from build123d import *
from build123d.topology import SkipClean

# Parameters (mm, degrees)
SKETCH_1_W          = 50
SKETCH_1_H          = 15
SKETCH_1_R          = 1.1
SKETCH_1_R_2        = 1.5
SKETCH_1_R_3        = 2.6
EXTRUDE_1_DEPTH     = 2
SKETCH_3_R          = 3
CUT_EXTRUDE_1_DEPTH = 1.5
SKETCH_1_7_W        = 17
SKETCH_1_7_H        = 15
SKETCH_1_7_R        = 1.5
SKETCH_1_7_R_2      = 1.1
EXTRUDE_4_DEPTH     = 4
SKETCH_1_8_R        = 6
SKETCH_1_8_R_2      = 1.5
SKETCH_1_8_R_3      = 1.1
CUT_EXTRUDE_4_DEPTH = 2
CUT_EXTRUDE_5_DEPTH = 15
EXTRUDE_START       = 2
SKETCH_8_R          = 5.5
SKETCH_8_R_2        = 2.6
EXTRUDE_11_DEPTH    = 2
CUT_EXTRUDE_6_DEPTH = 3.5
CUT_EXTRUDE_7_DEPTH = 2
FILLET_1_R          = 2
EXTRUDE_15_DEPTH    = 1
EXTRUDE_16_DEPTH    = 2
SKETCH_16_R         = 4.1
SKETCH_16_R_2       = 2.6
EXTRUDE_18_DEPTH    = 5
FILLET_3_R          = 0.5


with BuildPart() as part:
    # 草图1 → 凸台-拉伸1 (new body)
    with BuildSketch(Plane(origin=(0, 0, 0), x_dir=(1, 0, 0), z_dir=(0, 1, 0))):
        Rectangle(SKETCH_1_W, SKETCH_1_H)
        with BuildLine():
            ThreePointArc((8, 2.598076211), (8.5, 0), (8, -2.598076211))
            Line((8, -2.598076211), (8, 2.598076211))
        make_face(mode=Mode.SUBTRACT)
        with Locations(Location((-19.330127019, -2.5, 0), (0, 0, 270))):
            Circle(SKETCH_1_R, mode=Mode.SUBTRACT)
        with Locations(Location((-15, 0, 0), (0, 0, 270))):
            Circle(SKETCH_1_R_2, mode=Mode.SUBTRACT)
        with Locations(Location((-10.669872981, 2.5, 0), (0, 0, 270))):
            Circle(SKETCH_1_R, mode=Mode.SUBTRACT)
        with Locations(Location((1.5, 0, 0), (0, 0, 270))):
            Circle(SKETCH_1_R_3, mode=Mode.SUBTRACT)
        with Locations(Location((17.5, 3.5, 0), (0, 0, 270))):
            Circle(SKETCH_1_R, mode=Mode.SUBTRACT)
        with Locations(Location((17.5, -3.5, 0), (0, 0, 270))):
            Circle(SKETCH_1_R, mode=Mode.SUBTRACT)
        with Locations(Location((14, 0, 0), (0, 0, 270))):
            Circle(SKETCH_1_R, mode=Mode.SUBTRACT)
        with Locations(Location((17.5, 0, 0), (0, 0, 270))):
            Circle(SKETCH_1_R_2, mode=Mode.SUBTRACT)
        with Locations(Location((21, 0, 0), (0, 0, 270))):
            Circle(SKETCH_1_R, mode=Mode.SUBTRACT)
    extrude(amount=EXTRUDE_1_DEPTH)

    # 草图3 → 切除-拉伸1 (cut)
    with BuildSketch(Plane.XZ):
        with Locations(Location((-15, 0, 0), (0, 0, 270))):
            Circle(SKETCH_3_R)
    extrude(amount=-CUT_EXTRUDE_1_DEPTH, mode=Mode.SUBTRACT)

    # 草图1<7> → 凸台-拉伸4 (add)
    with BuildSketch(Plane(origin=(0, 0, 0), x_dir=(1, 0, 0), z_dir=(0, 1, 0))):
        with Locations((16.5, 0)):
            Rectangle(SKETCH_1_7_W, SKETCH_1_7_H)
        with Locations(Location((17.5, 0, 0), (0, 0, 270))):
            Circle(SKETCH_1_7_R, mode=Mode.SUBTRACT)
        with Locations(Location((21, 0, 0), (0, 0, 270))):
            Circle(SKETCH_1_7_R_2, mode=Mode.SUBTRACT)
        with Locations(Location((17.5, -3.5, 0), (0, 0, 270))):
            Circle(SKETCH_1_7_R_2, mode=Mode.SUBTRACT)
        with Locations(Location((14, 0, 0), (0, 0, 270))):
            Circle(SKETCH_1_7_R_2, mode=Mode.SUBTRACT)
        with Locations(Location((17.5, 3.5, 0), (0, 0, 270))):
            Circle(SKETCH_1_7_R_2, mode=Mode.SUBTRACT)
    extrude(amount=EXTRUDE_4_DEPTH)

    # 草图1<8> → 切除-拉伸4 (cut)
    with BuildSketch(Plane(origin=(0, 0, 0), x_dir=(1, 0, 0), z_dir=(0, 1, 0))):
        with Locations(Location((17.5, 0, 0), (0, 0, 270))):
            Circle(SKETCH_1_8_R)
        with Locations(Location((17.5, 0, 0), (0, 0, 270))):
            Circle(SKETCH_1_8_R_2, mode=Mode.SUBTRACT)
        with Locations(Location((21, 0, 0), (0, 0, 270))):
            Circle(SKETCH_1_8_R_3, mode=Mode.SUBTRACT)
        with Locations(Location((17.5, -3.5, 0), (0, 0, 270))):
            Circle(SKETCH_1_8_R_3, mode=Mode.SUBTRACT)
        with Locations(Location((14, 0, 0), (0, 0, 270))):
            Circle(SKETCH_1_8_R_3, mode=Mode.SUBTRACT)
        with Locations(Location((17.5, 3.5, 0), (0, 0, 270))):
            Circle(SKETCH_1_8_R_3, mode=Mode.SUBTRACT)
    extrude(amount=CUT_EXTRUDE_4_DEPTH, mode=Mode.SUBTRACT)

    # 草图6 → 切除-拉伸5 (cut)
    with BuildSketch(Plane(origin=(0, 0, -7.5), x_dir=(-1, 0, 0), z_dir=(0, 0, -1))):
        Polygon((-8, 2), (-11.464101615, 4), (-8, 4), align=None)
    extrude(amount=-CUT_EXTRUDE_5_DEPTH, mode=Mode.SUBTRACT)

    # 草图8 → 凸台-拉伸11 (add)
    with SkipClean():  # the faces are left unmerged after this step: merging them gives an invalid solid
        with BuildSketch(Plane.XZ.offset(EXTRUDE_START)):
            with Locations(Location((1.5, 0, 0), (0, 0, 90))):
                Circle(SKETCH_8_R)
            with Locations(Location((1.5, 0, 0), (0, 0, 270))):
                Circle(SKETCH_8_R_2, mode=Mode.SUBTRACT)
        extrude(amount=-EXTRUDE_11_DEPTH)

    # 草图10 → 切除-拉伸6 (cut)
    with BuildSketch(Plane.XZ.offset(2)):
        Polygon((1.5, 3.175426481), (-1.25, 1.58771324), (-1.25, -1.58771324), (1.5, -3.175426481), (4.25, -1.58771324), (4.25, 1.58771324), align=None)
    extrude(amount=-CUT_EXTRUDE_6_DEPTH, mode=Mode.SUBTRACT)

    # 草图11 → 切除-拉伸7 (cut)
    with BuildSketch(Plane.XZ.offset(2)):
        with BuildLine():
            Line((-3.398979486, 2.5), (6.398979486, 2.5))
            ThreePointArc((6.398979486, 2.5), (1.5, 5.5), (-3.398979486, 2.5))
        make_face()
    extrude(amount=-CUT_EXTRUDE_7_DEPTH, mode=Mode.SUBTRACT)

    # 圆角1
    fillet_1_edges = [part.edges().sort_by_distance(p)[0] for p in [
        (-25, 1, -7.5),
        (25, 2, -7.5),
    ]]
    fillet(fillet_1_edges, radius=FILLET_1_R)

    # 草图13 → 凸台-拉伸15 (add)
    with BuildSketch(Plane.XY.offset(7.5)):
        Polygon((11.464101615, 4), (8, 2), (-25, 2), (-25, 0), (25, 0), (25, 4), align=None)
    extrude(amount=EXTRUDE_15_DEPTH)

    # 草图14 → 凸台-拉伸16 (add)
    with BuildSketch(Plane.XY.offset(8.5)):
        Polygon((8, 0), (8, 2), (11.464101615, 4), (25, 4), (25, 0), align=None)
    extrude(amount=EXTRUDE_16_DEPTH)

    # 草图16 → 凸台-拉伸18 (add)
    with BuildSketch(Plane(origin=(0, 2, 0), x_dir=(1, 0, 0), z_dir=(0, 1, 0))):
        with Locations(Location((1.5, 0, 0), (0, 0, 270))):
            Circle(SKETCH_16_R)
        with Locations(Location((1.5, 0, 0), (0, 0, 90))):
            Circle(SKETCH_16_R_2, mode=Mode.SUBTRACT)
    extrude(amount=EXTRUDE_18_DEPTH)

    # 圆角3
    fillet_3_edges = [part.edges().sort_by_distance(p)[0] for p in [
        (4.25, -2, 0),
        (3.459936491, -2, 2.04385662),
        (-1.25, -2, 0),
        (0.125, -2, -2.38156986),
        (2.875, -2, -2.38156986),
        (-0.459936491, -2, 2.04385662),
        (1.5, -2, -5.5),
        (4.534426233, -2, 2.5),
        (-1.534426233, -2, 2.5),
    ]]
    fillet(fillet_3_edges, radius=FILLET_3_R)


solid = part.part
Verification items for the finished model (mm, model axes). A direction names the side the tool comes from. Give positions to 0.01 mm unless a question says otherwise; leave off trailing zeros. Loops run counter-clockwise (first coordinate to the right, second up) from the corner with the lowest first, then second, coordinate; pieces in that order, holes last.
1) Depth check by flat-ended pin: pin 1 Ø1 at (x, z) = (1.5, 2.5) entering from -Y; pin 2 Ø3.5 at (x, z) = (17.5, 0) entering from -Y; pin 3 Ø5 at (x, y) = (-18.5, 0.5) entering from +Z. Enter the tip coordinate at first touch or a pass-through.
2) Thickness scan on line 1 along X through (y, z) = (1.1, 0); line 2 along X through (y, z) = (1.6, 0); line 3 along X through (y, z) = (0.75, -5.5). Record the ranges inside material, lowest first.
3) Set-up check for faces 1 (the cylindrical face through (-11.646, 0.986, -1.992)), 2 (the flat face through (-9, 1, 8.5)), 3 (the cylindrical face through (0.073, -1.857, -2.525)): record each of +Z, -Z, +X, -X, +Y, -Y from which the full face is reachable in a straight line by a thin tool's end or side.
4) Sectioned sample at D-D, the plane y = 5.5. Enter the section's corners in (x, z).
5) Draft check along Z on faces 4 (the flat face through (4.25, 0, 0)), 5 (the flat face through (4.8, 1.5, -7.5)), 6 (the flat face through (20, 4, 1)), 7 (the flat face through (-2, -1, 2.5)). Enter one of: pulls with the +Z half, pulls with the -Z half, needs draft (parallel to the pull), parting line crosses it, or undercut.
6) Sectioned sample at A-A, the plane x = 14. Enter the section's corners in (y, z).
7) Sectioned sample at B-B, the plane y = -1. Enter the section's corners in (x, z).
8) Sectioned sample at C-C, the plane z = 9. Enter the section's corners in (x, y).
Answers:
1. pin 1: stops at y = 1.5
1. pin 2: stops at y = 2
1. pin 3: stops at z = 8.5
2. line 1: x = -25 to -18, -12 to -1.25, 4.25 to 11.5, 23.5 to 25
2. line 2: x = -25 to -16.5, -13.5 to -1.1, 4.1 to 11.5, 23.5 to 25
2. line 3: x = -25 to 15.1, 19.9 to 25
3. face 1: +Y, -Y
3. face 2: +Z, -X, +Y, -Y
3. face 3: -Y
4. outline: circle Ø8.2 at (1.5, 0); hole circle Ø5.2 at (1.5, 0)
5. face 4: undercut
5. face 5: pulls with the -Z half
5. face 6: needs draft
5. face 7: pulls with the +Z half
6. outline: (0, -7.5) - (4, -7.5) - (4, -1.1) - (2, -1.1) - (2, -4.87) - (0, -4.87) - close; (0, 4.87) - (2, 4.87) - (2, 1.1) - (4, 1.1) - (4, 10.5) - (0, 10.5) - close
7. outline: (-3.4, 2.5) arc R5.5 ccw (long way) to (6.4, 2.5) - (2.67, 2.5) - (4.25, 1.59) - (4.25, -1.59) - (1.5, -3.18) - (-1.25, -1.59) - (-1.25, 1.59) - (0.33, 2.5) - close
8. outline: (8, 0) - (25, 0) - (25, 4) - (11.46, 4) - (8, 2) - close
